Verification items for the finished model (mm, model axes). A direction names the side the tool comes from. Coordinates: 2 decimals unless noted, no trailing zeros. Order: outer loops, then holes, each group sorted by start corner. A loop starts at its lowest first (then second) coordinate and runs counter-clockwise, first axis right, second up. Notation, with made-up numbers: M -31.5,75 L 4.5,75 A29 cw 4.5,101 Z; hole C 21,81.25 d2. An arc over 180 degrees is marked long. Answer as a JSON object with one key per item and string values. Group by question number.
(1) Material ranges on line 1 (X direction, y = 2, z = 45); line 2 (Z direction, x = 21.5, y = 8.5); line 3 (Z direction, x = 17.5, y = 12.5), recorded low to high.
(2) Gauge pin test, flat ends, axial feed: pin 1 Ø5 at (x, z) = (18, -6) entering from -Y; pin 2 Ø10 at (y, z) = (-3.5, 16.5) entering from +X; pin 3 Ø1.5 at (x, y) = (28, -1) entering from +Z. Record the tip position at first contact, or that the pin passes through.
(3) Cross-section at A-A (x = 23). Count the separate pieces of the cut face and the enclosed holes in it, plus the area to 3 significant figures.
(4) Mould release check, pull along Y, two halves, no side actions. Record for faces 6 (the face through (27.931, 16.366, 41.037)), 7 (the face through (23.64, 11.23, 39.95)), 8 (the face through (10.984, 3.496, 8.426)), 9 (the face through (7.955, -6.796, 39.947)): released by +Y, released by -Y, zero draft, split by the parting line, or undercut.
(5) Cross-section at C-C (z = 6.5). Enter the section's corners in (x, y).
(6) Access from +Z, -Z, +X, -X, +Y, -Y to the whole of each face (thin tool, end or side, straight path). Record for faces 1 (the face through (23.64, -6.97, 39.95)), 2 (the face through (0, 2, 41)), 3 (the face through (12, 7, -31.05)), 4 (the face through (1.81, 2.06, 17.85)), 5 (the face through (15.831, 18.176, 17.849)).
(7) Cross-section at B-B (z = -29). Enter the section's corners in (x, y).
from build123d import *

# Parameters (mm, degrees)
F0_W        = 35.713232588
F0_H        = 43.3274284005
F1_DEPTH    = 31.75
F2_T        = -5.08
F3_R        = 12.7
F4_T1_DEPTH = 38.2474284005
F5_R        = 6.35
F6_R        = 5.07999
F7_R        = 4.4336766497
F8_DEPTH    = 15.24
F9_R        = 8.453024689
F10_DEPTH   = 5.08
F11_R       = 5.07999
F12_R       = 4.45495875
F13_DEPTH   = 3.81
F14_R       = 11.3706075555
F15_DEPTH   = 6.35
F16_R       = 5.08
F17_R       = 4.5498563982
F18_DEPTH   = 16.51
F19_R       = 14.5872026809
F20_DEPTH   = 5.08


# Not quite as in the source:
# - a fillet or chamfer that OpenCascade refuses, or shapes differently, is made with other operations: its cross-section is extruded or revolved along the edge and cut away or added
# - a fillet or chamfer is up to 0.001 mm smaller than in the source, because OpenCascade refuses the exact size


with BuildPart() as f1:
    # F0 (on Right) → F1 (new body)
    with BuildSketch(Plane.YZ):
        with Locations((2.1306423005, 37.6035124063)):
            Rectangle(F0_W, F0_H)
    extrude(amount=F1_DEPTH)

    # F2
    f2_openings = [f1.faces().sort_by_distance(p)[0] for p in [
        (15.875, 2.130642, 59.267227),
    ]]
    offset(amount=F2_T, openings=f2_openings)

    # F3
    f3_edges = [f1.edges().sort_by_distance(p)[0] for p in [
        (0, -15.725974, 37.603512),
        (31.75, -15.725974, 37.603512),
        (31.75, 19.987259, 37.603512),
        (0, 19.987259, 37.603512),
    ]]
    fillet(f3_edges, radius=F3_R)

    # F4: fillet of radius 11.43 on 4 edges, made by hand

    # F4_s2 → F4_t1 (join)
    with BuildSketch(Plane.XY.offset(21.0197982061)):
        with BuildLine():
            ThreePointArc((5.08, 0.7840260065), (8.427769491, -7.2982045025), (16.51, -10.6459739935))
            Line((16.51, -10.6459739935), (5.08, -10.6459739935))
            Line((5.08, -10.6459739935), (5.08, 0.7840260065))
        make_face()
        with BuildLine():
            ThreePointArc((16.51, 14.9072585945), (8.427769491, 11.5594891034), (5.08, 3.4772585945))
            Line((5.08, 3.4772585945), (5.08, 14.9072585945))
            Line((5.08, 14.9072585945), (16.51, 14.9072585945))
        make_face()
        with BuildLine():
            ThreePointArc((15.24, 14.9072585945), (23.322230509, 11.5594891034), (26.67, 3.4772585945))
            Line((26.67, 3.4772585945), (26.67, 14.9072585945))
            Line((26.67, 14.9072585945), (15.24, 14.9072585945))
        make_face()
        with BuildLine():
            ThreePointArc((15.24, -10.6459739935), (23.322230509, -7.2982045025), (26.67, 0.7840260065))
            Line((26.67, 0.7840260065), (26.67, -10.6459739935))
            Line((26.67, -10.6459739935), (15.24, -10.6459739935))
        make_face()
    extrude(amount=F4_T1_DEPTH)

    # F5
    f5_edges = [f1.edges().sort_by_distance(p)[0] for p in [
        (15.875, -15.725974, 15.939798),
        (3.719744, -12.00623, 15.939798),
        (0, 2.130642, 15.939798),
        (3.719744, 16.267515, 15.939798),
        (15.875, 19.987259, 15.939798),
        (28.030256, 16.267515, 15.939798),
        (31.75, 2.130642, 15.939798),
        (28.030256, -12.00623, 15.939798),
    ]]
    fillet(f5_edges, radius=F5_R)

    # F6 (radius 5.08 in the source; OpenCascade refuses exactly that, so slightly less here)
    f6_edges = [f1.edges().sort_by_distance(p)[0] for p in [
        (15.875, 14.889606, 40.143512),
        (26.67, 3.477259, 40.143512),
        (23.543702, 11.331775, 21.019798),
        (23.543702, 11.331775, 59.267227),
        (15.875, -10.628321, 40.143512),
        (26.67, 0.784026, 40.143512),
        (23.543702, -7.07049, 21.019798),
        (23.543702, -7.07049, 59.267227),
        (5.08, 3.477259, 40.143512),
        (8.206298, 11.331775, 21.019798),
        (8.206298, 11.331775, 59.267227),
        (5.08, 0.784026, 40.143512),
        (8.206298, -7.07049, 21.019798),
        (8.206298, -7.07049, 59.267227),
    ]]
    fillet(f6_edges, radius=F6_R)

    # F7 (on face) → F8 (join)
    with BuildSketch(Plane(origin=(0, 0, 15.9397982061), x_dir=(1, 0, 0), z_dir=(0, 0, -1))):
        with Locations((15.4130682349, -3.6905435845)):
            Circle(F7_R)
    extrude(amount=F8_DEPTH)

    # F9 (on face) → F10 (join)
    with BuildSketch(Plane(origin=(0, 0, 0.6997982061), x_dir=(1, 0, 0), z_dir=(0, 0, -1))):
        with Locations((15.4130682349, -3.6905435845)):
            Circle(F9_R)
    extrude(amount=F10_DEPTH)

    # F11 (radius 5.08 in the source; OpenCascade refuses exactly that, so slightly less here)
    f11_edges = [f1.edges().sort_by_distance(p)[0] for p in [
        (6.960044, 3.690544, -4.380202),
    ]]
    fillet(f11_edges, radius=F11_R)

    # F12 (on face) → F13 (join)
    with BuildSketch(Plane(origin=(0, 0, -4.3802017939), x_dir=(1, 0, 0), z_dir=(0, 0, -1))):
        with Locations((15.4130682349, -3.6905435845)):
            Circle(F12_R)
    extrude(amount=F13_DEPTH)

    # F14 (on face) → F15 (join)
    with BuildSketch(Plane(origin=(0, 0, -8.1902017939), x_dir=(1, 0, 0), z_dir=(0, 0, -1))):
        with Locations((15.4130682349, -3.6905435845)):
            Circle(F14_R)
    extrude(amount=F15_DEPTH)

    # F16
    f16_edges = [f1.edges().sort_by_distance(p)[0] for p in [
        (4.042461, 3.690544, -14.540202),
    ]]
    fillet(f16_edges, radius=F16_R)

    # F17 (on face) → F18 (join)
    with BuildSketch(Plane(origin=(0, 0, -14.5402017939), x_dir=(1, 0, 0), z_dir=(0, 0, -1))):
        with Locations((15.4130682349, -3.6905435845)):
            Circle(F17_R)
    extrude(amount=F18_DEPTH)

    # F19 (on face) → F20 (join)
    with BuildSketch(Plane(origin=(0, 0, -31.0502017939), x_dir=(1, 0, 0), z_dir=(0, 0, -1))):
        with Locations((15.4130682349, -3.6905435845)):
            Circle(F19_R)
    extrude(amount=F20_DEPTH)


solid = f1.part
Taken from the geometry:
{
 "1": {"line 1": "x = 0 to 5.08, 26.67 to 31.75", "line 2": "z = -36.13 to -31.05, -14.32 to -8.19, -1.87 to 0.7, 15.94 to 21.3", "line 3": "z = -36.13 to -31.05, -13.72 to -8.19, 15.94 to 21.97"},
 "2": {"pin 1": "stops at y = -7.6", "pin 2": "stops at x = 31.7", "pin 3": "stops at z = 58.37"},
 "3": {"separate pieces": "4", "enclosed holes": "0", "area": "967 mm²"},
 "4": {"face 6": "released by +Y", "face 7": "undercut", "face 8": "split by the parting line", "face 9": "undercut"},
 "5": {"outline": "C 15.41,3.69 d8.87"},
 "6": {"face 1": "+Z", "face 2": "+Z, -Z, -X, +Y, -Y", "face 3": "none", "face 4": "-X, +Y, -Y", "face 5": "+X, -X, +Y"},
 "7": {"outline": "C 15.41,3.69 d9.1"}
}
